The drawing under review shows one solid part. Ordinate dimensions are in mm from its lowest x, y, z. A direction names the side the tool comes from. Coordinates: 2 decimals unless noted, no trailing zeros. Write each loop counter-clockwise with the first axis right and the second up, starting at its lowest first coordinate (ties: lowest second). Pieces come first, ordered by that corner, then holes.
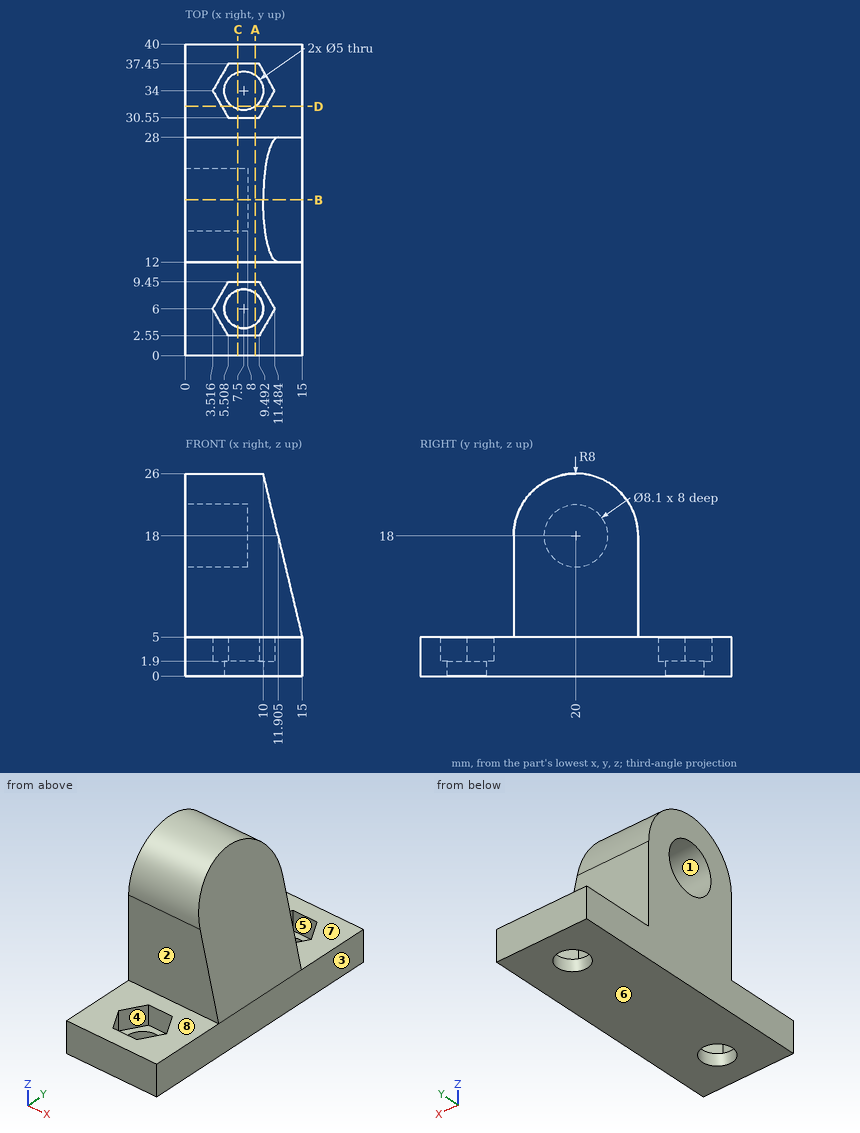
Q1. Add section B-B (y = 20). State the section outline as (x, z) points, then the cut area to 3 significant figures.
Ans:
outline: (0, 0) - (15, 0) - (15, 5) - (10, 26) - (0, 26) - (0, 22.05) - (8, 22.05) - (8, 13.95) - (0, 13.95) - close
area: 273 mm2
Q2. For probe 1 along X at (y, z) = (34, 0.95); probe 2 along Z at (x, y) = (6.25, 20); probe 3 along Z at (x, y) = (9.25, 11.5), list the stretches that pass through material, from the lowest coordinate up.
Ans:
probe 1: x = 0 to 5, 10 to 15
probe 2: z = 0 to 13.95, 22.05 to 26
probe 3: z = 0 to 5
Q3. Draft analysis for pull direction Y (two halves, no side actions). For the marked faces 1, 2, 3 and 4, state which applies: +Y half, -Y half, draft (parallel to the pull), parting line (faces both ways), or undercut.
Ans:
face 1: undercut
face 2: -Y half
face 3: draft
face 4: undercut
Q4. Tool access review of the marked faces 5, 6, 7 and 8: name each direction out of +Z, -Z, +X, -X, +Y, -Y from which nothing blocks a thin tool from reaching the whole face with its end or side.
Ans:
face 5: +Z
face 6: -Z, +X, -X, +Y, -Y
face 7: +Z, +X, -X, +Y
face 8: +Z, +X, -X, -Y
Q5. Add section C-C (x = 6.75). Give the number of separate pieces and of enclosed holes in the cut face, then the cut area to 3 significant figures.
Ans:
separate pieces: 3
enclosed holes: 1
area: 396 mm2
Q6. Add section A-A (x = 9). State the section outline as (y, z) points.
Ans:
outline: (0, 0) - (4, 0) - (4, 1.9) - (2.55, 1.9) - (2.55, 5) - (0, 5) - close; (8, 0) - (32, 0) - (32, 1.9) - (30.55, 1.9) - (30.55, 5) - (28, 5) - (28, 18) arc R8 ccw to (12, 18) - (12, 5) - (9.45, 5) - (9.45, 1.9) - (8, 1.9) - close; (36, 0) - (40, 0) - (40, 5) - (37.45, 5) - (37.45, 1.9) - (36, 1.9) - close
Q7. Add section D-D (y = 32). State the section outline as (x, z) points.
Ans:
outline: (0, 0) - (6, 0) - (6, 1.9) - (4.67, 1.9) - (4.67, 5) - (0, 5) - close; (9, 0) - (15, 0) - (15, 5) - (10.33, 5) - (10.33, 1.9) - (9, 1.9) - close
Q8. Clearance check with flat-ended pins moving along their axes: pin 1 Ø6 at (x, y) = (7.5, 34) entering from +Z; pin 2 Ø5.5 at (x, y) = (7.5, 32.5) entering from +Z; pin 3 Ø6 at (x, y) = (3.5, 24) entering from +Z; pin 4 Ø1.5 at (x, y) = (4.5, 19.5) entering from +Z. State where each tip first meets the part, or that it passes through.
Ans:
pin 1: stops at z = 1.9
pin 2: stops at z = 5
pin 3: stops at z = 25.94
pin 4: stops at z = 26
